Read the model definition and answer for the solid it produces. Units are mm, in the model's axes. Give positions to 0.01 mm unless a question says otherwise; leave off trailing zeros. Write each loop counter-clockwise with the first axis right and the second up, starting at its lowest first coordinate (ties: lowest second). Pieces come first, ordered by that corner, then holes. Notation, with made-up numbers: M 51,54 L 103,54 A16 ccw 103,72 Z; hole C 72.25,-32.75 d10. An arc over 180 degrees is marked long. Use a Markdown table: item, result. Add a question column.
Item 1: Consider probe 1 along Z at (x, y) = (0, 2.25); probe 2 along Z at (x, y) = (15.5, -3.5); probe 3 along X at (y, z) = (-2.75, -27). Determine where each line is inside the solid, lowest interval first. Write a range as [from, to].
Item 2: Given P1, Ø8, axis at x = -18, z = 23.5, coming from the -Y side; P2, Ø4, axis at x = 6, y = -1, coming from the +Z side; P3, Ø4, axis at y = 0, z = 3, coming from the -X side; P4, Ø21, axis at x = -14, z = -4.5, coming from the +Y side, each flat-ended and moving along its own axis, determine where each tip first touches the part or whether it passes through.
Item 3: A cutting plane is placed at A-A on y = -2.25. Determine the outline of the cut face in (x, z).
Item 4: The mould has two halves that part along Z. Classify faces 1 (the cylindrical face through (17.535, -0.049, -33.713)), 2 (the flat face through (-25.9, 4, -16.4)), 3 (the cylindrical face through (-29.97, 0.05, 1.32)): pulls with the +Z half, pulls with the -Z half, needs draft (parallel to the pull), parting line crosses it, or undercut.
from build123d import *

# Parameters (mm, degrees)
CHAMFER_1_SIZE = 0.5


with BuildPart() as part:
    # 草图1 → 旋转1 (revolve)
    with BuildSketch(Plane.XY):
        Polygon((30, -4), (30, 4), (32, 4), (32, 3.8), (32.2, 3.8), (32.2, 4), (35.1, 4), (35.1, 3.8), (35.2, 3.8), (35.2, 4), (38, 4), (38, -4), (35.2, -4), (35.2, -3.8), (35.1, -3.8), (35.1, -4), (32.2, -4), (32.2, -3.8), (32, -3.8), (32, -4), align=None)
    revolve(axis=Axis((0, 60.459632728, 0), (0, -1, 0)))

    # 倒角1
    chamfer_1_edges = [part.edges().sort_by_distance(p)[0] for p in [
        (-38, 4, 0),
        (-38, -4, 0),
        (-30, -4, 0),
        (-30, 4, 0),
    ]]
    chamfer(chamfer_1_edges, length=CHAMFER_1_SIZE)


solid = part.part
Filled in:
| question | item | result |
|---|---|---|
| 1 | probe 1 | [-38, -30], [30, 38] |
| 1 | probe 2 | [-34.7, -25.69], [25.69, 34.7] |
| 1 | probe 3 | [-26.74, -13.08], [13.08, 26.74] |
| 2 | P1 | y = -4 |
| 2 | P2 | z = 37.79 |
| 2 | P3 | x = -37.99 |
| 2 | P4 | through |
| 3 | outline | C 0,0 d76; hole C 0,0 d60 |
| 4 | face 1 | parting line crosses it |
| 4 | face 2 | needs draft |
| 4 | face 3 | undercut |
